Verification items for the finished model (mm, model axes). A direction names the side the tool comes from. Give positions to 0.01 mm unless a question says otherwise; leave off trailing zeros. Loops run counter-clockwise (first coordinate to the right, second up) from the corner with the lowest first, then second, coordinate; pieces in that order, holes last. Notation, with made-up numbers: M 40,72.5 L 51,72.5 A12 ccw 51,82.5 Z; hole C 19,11.25 d11. An arc over 180 degrees is marked long. Use CSV: the item, a comma, the result in double quotes.
Autodesk Inventor part; units mm, degrees
ref_plane "Arbeitsebene3" through (-10.5, -12.5, -1.5) normal (0, 0, -1) x (0, 1, 0)
ref_plane "YZ Plane" through (0, 0, 0) normal (1, 0, 0) x (0, 1, 0)
ref_plane "XZ Plane" through (0, 0, 0) normal (0, 1, 0) x (-1, 0, 0)
ref_plane "Arbeitsebene1" through (0, 0, 0) normal (0, 0, 1) x (1, 0, 0)
ref_plane "Arbeitsebene2" through (-2.35, 3.95, -7.1) normal (0, 0, -1) x (-1, 0, 0)
sketch "Skizze1" plane through (-2.35, 3.95, -7.1) normal (0, 0, -1) x (-1, 0, 0)
  line L0 (7.75, 3.25) -> (7.75, -3.25)
  line L1 (7.75, -3.25) -> (2.75, -3.25)
  line L2 (2.75, -3.25) -> (2.75, 3.25)
  line L3 (2.75, 3.25) -> (7.75, 3.25)
  line L4 (9.25, -6.8) -> (9.25, 6.8)
  line L5 (9.25, 6.8) -> (-9.25, 6.8)
  line L6 (-9.25, 6.8) -> (-9.25, -6.8)
  line L7 (-9.25, -6.8) -> (9.25, -6.8)
  line L8 (14.25, 9.8) -> (-21.25, 9.8)
  line L9 (-21.25, 9.8) -> (-21.25, -10.8)
  line L10 (-21.25, -10.8) -> (14.25, -10.8)
  line L11 (14.25, -10.8) -> (14.25, 9.8)
  point P0 (-2.35, -3.95)
  dimension "d0" = 5
  dimension "d1" = 3
  dimension "d2" = 4
  dimension "d3" = 12
extrude "Extrusion1" add sketch "Skizze1" along normal blind 6 contours L7 L6 L5 L4 | L11 L10 L9 L8
sketch "Skizze2" plane through (-2.35, 3.95, -7.1) normal (0, 0, 1) x (1, 0, 0)
  line L0 (-9.25, -6.8) -> (-9.25, 6.8)
  line L1 (9.25, -6.8) -> (-9.25, -6.8)
  line L2 (9.25, 6.8) -> (9.25, -6.8)
  line L3 (-9.25, 6.8) -> (9.25, 6.8)
  line L4 (9.55, 7.1) -> (9.55, -7.1)
  line L5 (9.55, -7.1) -> (-9.55, -7.1)
  line L6 (-9.55, -7.1) -> (-9.55, 7.1)
  line L7 (-9.55, 7.1) -> (9.55, 7.1)
  line L8 (21.25, 9.8) -> (21.25, -10.8)
  line L9 (-14.25, 9.8) -> (21.25, 9.8)
  line L10 (-14.25, -10.8) -> (-14.25, 9.8)
  line L11 (21.25, -10.8) -> (-14.25, -10.8)
  line L12 (-7.75, 3.25) -> (-7.75, -3.25)
  line L13 (-2.75, 3.25) -> (-7.75, 3.25)
  line L14 (-2.75, -3.25) -> (-2.75, 3.25)
  line L15 (-7.75, -3.25) -> (-2.75, -3.25)
  point P0 (2.35, -3.95)
  dimension "d6" = 0.3
ref_plane "Arbeitsebene3" through (-10.5, -12.5, -1.5) normal (0, 0, -1) x (0, 1, 0)
extrude "Extrusion2" add sketch "Skizze2" along normal up to surface (5.6 mm away) contours L8 L11 L10 L9
sketch "Skizze3" plane through (-16.6, 13.75, -1.5) normal (0, 0, 1) x (1, 0, 0)
  line L0 (23.5, -26.25) -> (23.5, -1.25)
  line L1 (23.5, -1.25) -> (6.1, -1.25)
  line L2 (6.1, -1.25) -> (6.1, -26.25)
  line L3 (6.1, -26.25) -> (23.5, -26.25)
  line L4 (24.5, -27.25) -> (24.5, -0.25)
  line L5 (24.5, -0.25) -> (5.1, -0.25)
  line L6 (5.1, -0.25) -> (5.1, -27.25)
  line L7 (5.1, -27.25) -> (24.5, -27.25)
  line L8 (4.7, -2.7) -> (23.8, -2.7)
  line L9 (23.8, -2.7) -> (23.8, -16.9)
  line L10 (23.8, -16.9) -> (4.7, -16.9)
  line L11 (4.7, -16.9) -> (4.7, -2.7)
  line L12 (35.5, 0) -> (0, 0)
  line L13 (0, 0) -> (0, -20.6)
  line L14 (0, -20.6) -> (35.5, -20.6)
  line L15 (35.5, -20.6) -> (35.5, 0)
  point P0 (16.6, -13.75)
  point P1 (24.5, -20.6)
  point P2 (5.1, -20.6)
  point P3 (5.1, -16.9)
  point P4 (5.1, -2.7)
  dimension "d9" = 1
extrude "Extrusion3" add sketch "Skizze3" along normal blind 5.5 contours L4 L5 L6 L8 L11 L10 L14 L13 L12 L15
sketch "Skizze4" plane through (18.9, -6.85, -13.1) normal (1, 0, 0) x (0, 0, -1)
  circle A0 centre (-8.8, 10.8) radius 6.75
  circle A1 centre (-8.8, 10.8) radius 6.5405
  point P0 (-13.1, 6.85)
  dimension "d30" = 13.5
extrude "Extrusion4" cut sketch "Skizze4" against normal blind 10.5 contours A0 | A1
sketch "Skizze5" plane through (8.4, -6.85, -13.1) normal (1, 0, 0) x (0, 0, -1)
  circle A0 centre (-8.8, 10.8) radius 4.5085
  point P0 (-13.1, 6.85)
extrude "Extrusion5" cut sketch "Skizze5" against normal blind 6
sketch "Skizze6" plane through (-16.6, -6.85, -13.1) normal (0, -1, 0) x (1, 0, 0)
  line L0 (0, 17.1) -> (0, 0)
  line L1 (35.5, 0) -> (0, 0)
  line L2 (35.5, 17.1) -> (35.5, 0)
  line L3 (24.5, 17.1) -> (35.5, 17.1)
  line L4 (24.5, 11.6) -> (24.5, 17.1)
  line L5 (5.1, 11.6) -> (24.5, 11.6)
  line L6 (5.1, 11.6) -> (5.1, 17.1)
  line L7 (0, 17.1) -> (5.1, 17.1)
  line L8 (11.5, 6) -> (11.5, 0)
  line L9 (35.5, 0) -> (15.5, 0)
  line L10 (15.5, 0) -> (15.5, -10)
  line L11 (15.5, -10) -> (35.5, -10)
  line L12 (35.5, -10) -> (35.5, 0)
  line L13 (30.4199, -5) -> (20.5801, -5) construction
  line L14 (30.4199, -3) -> (20.5801, -3)
  line L15 (20.5801, -7) -> (30.4199, -7)
  arc A0 (30.4199, -7) -> (30.4199, -3) centre (30.4199, -5) ccw
  arc A1 (20.5801, -3) -> (20.5801, -7) centre (20.5801, -5) ccw
  point P0 (16.6, 13.1)
  point P1 (25.5, -5)
  dimension "d19" = 20
  dimension "d20" = 10
  dimension "d21" = 4
extrude "Extrusion6" add sketch "Skizze6" against normal up to surface (20.6 mm away) contours L1 L12 L11 L10
chamfer "Fase1" distance 5 angle 45 1 edges at (18.9, 3.95, 2.45)
chamfer "Fase2" distance 4 angle 45 4 edges at (-7.6, 0.7, -13.1) (-10.1, 3.95, -13.1) (-7.6, 7.2, -13.1) (-5.1, 3.95, -13.1)
properties part number "30_Scanlens_Laseradaper_v0"
(1) Scan lines: L1, parallel to Z at x = 5, y = -1.25; L2, parallel to Z at x = 7.15, y = 3.95; L3, parallel to Y at x = 12.55, z = -4.3. Record each from-to range of solid material in increasing order. Write a range as from..to.
Calculated:
L1,"z = -23.1..-20.1, -16.1..-7.1"
L2,"z = -23.1..-20.1, -16.1..-8.81"
L3,"y = -6.85..-2.8, 10.7..13.75"
(2) Depth check by flat-ended pin: pin 1 Ø1.2 at (y, z) = (11.5, 2) entering from +X; pin 2 Ø1 at (y, z) = (-1.5, -3) entering from +X; pin 3 Ø3.5 at (x, y) = (-1, -4.5) entering from +Z. Enter the tip coordinate at first touch or a pass-through.
Calculated:
pin 1,"stops at x = 17.58"
pin 2,"stops at x = 8.4"
pin 3,"stops at z = -1.5"
(3) Section check A-A on y = 3.95. Count the separate pieces of the cut face and the enclosed holes in it, plus the area to 3 significant figures.
Calculated:
separate pieces,"3"
enclosed holes,"1"
area,"315 mm²"
(4) Section check C-C on x = 9. Record the cut outline in (y, z), plus the area to 3 significant figures.
Calculated:
outline,"M -6.85,-23.1 L 13.75,-23.1 L 13.75,-20.1 L -6.85,-20.1 Z; M -6.85,-16.1 L 13.75,-16.1 L 13.75,4 L -6.85,4 Z; hole C 3.95,-4.3 d13.5"
area,"333 mm²"
(5) Tool access check on faces 1 (the cylindrical face through (6.081, 4.408, -8.785)), 2 (the flat face through (9, 3, -20.1)), 3 (the flat face through (-2.7, 3.8, -11.5)), 4 (the flat face through (-8, 0.7, -8)). Record the directions out of +Z, -Z, +X, -X, +Y, -Y that give a thin tool (end or side, any length) a straight path to the whole face; none if there is none.
Calculated:
face 1,"+X"
face 2,"+Y, -Y"
face 3,"-Z"
face 4,"+Z, -Z"
(6) Mould release check, pull along Y, two halves, no side actions. Record for faces 5 (the flat face through (1, 13.75, -6)), 6 (the flat face through (-7.7, -1.7, -11.5)), 7 (the flat face through (-16.6, 4, -5)): released by +Y, released by -Y, zero draft, split by the parting line, or undercut.
Calculated:
face 5,"released by +Y"
face 6,"undercut"
face 7,"zero draft"
(7) Section check B-B on z = -18.1. Record the cut outline in (x, y).
Calculated:
outline,"M -1.1,-6.85 L 1.98,-6.85 L 1.98,13.75 L -1.1,13.75 Z; M 15.82,-6.85 L 18.9,-6.85 L 18.9,13.75 L 15.82,13.75 Z"
(8) Section check D-D on z = -4.3. Record the cut outline in (x, y).
Calculated:
outline,"M -16.6,-6.85 L 17.95,-6.85 L 13.9,-2.8 L 8.4,-2.8 L 8.4,-0.56 L 7.2,-0.56 L 7.2,-3.15 L -11.9,-3.15 L -11.9,11.05 L 7.2,11.05 L 7.2,8.46 L 8.4,8.46 L 8.4,10.7 L 13.9,10.7 L 16.95,13.75 L -16.6,13.75 Z"
